from build123d import *

# Parameters (mm, degrees)
EXTRUDE_1_DEPTH     = 2
EXTRUDE_2_DEPTH     = 2
SKETCH_4_R          = 1
CUT_EXTRUDE_1_DEPTH = 2
EXTRUDE_4_DEPTH     = 2
SKETCH_8_R          = 1
CUT_EXTRUDE_3_DEPTH = 2


with BuildPart() as part:
    # 草图1 → 凸台-拉伸1 (new body)
    with BuildSketch(Plane.XY):
        Polygon((27.5, -11.5), (27.5, 11.5), (11.5, 11.5), (11.5, 27.5), (-11.5, 27.5), (-11.5, 11.5), (-27.5, 11.5), (-27.5, -11.5), (-11.5, -11.5), (-11.5, -27.5), (11.5, -27.5), (11.5, -11.5), align=None)
    extrude(amount=EXTRUDE_1_DEPTH)

    # 草图3 → 凸台-拉伸2 (add)
    with BuildSketch(Plane(origin=(0, 27.5, 0), x_dir=(1, 0, 0), z_dir=(0, 1, 0))):
        with BuildLine():
            Line((-11.5, -2), (11.5, -2))
            Line((11.5, -2), (11.5, 19.5))
            ThreePointArc((11.5, 19.5), (0, 31), (-11.5, 19.5))
            Line((-11.5, 19.5), (-11.5, -2))
        make_face()
    extrude_2 = extrude(amount=-EXTRUDE_2_DEPTH)

    # 草图4 → 切除-拉伸1 (cut)
    with BuildSketch(Plane(origin=(0, 27.5, 0), x_dir=(1, 0, 0), z_dir=(0, 1, 0))):
        with Locations((0, 19.5)):
            Circle(SKETCH_4_R)
    cut_extrude_1 = extrude(amount=-CUT_EXTRUDE_1_DEPTH, mode=Mode.SUBTRACT)

    # 镜向2: 凸台-拉伸2, 切除-拉伸1 across plane
    add(extrude_2.mirror(Plane.ZX))
    add(cut_extrude_1.mirror(Plane.ZX), mode=Mode.SUBTRACT)

    # 草图7 → 凸台-拉伸4 (add)
    with BuildSketch(Plane.ZY.offset(27.5)):
        with BuildLine():
            Line((0, 11.5), (21.5, 11.5))
            ThreePointArc((21.5, 11.5), (33, 0), (21.5, -11.5))
            Line((21.5, -11.5), (0, -11.5))
            Line((0, -11.5), (0, 11.5))
        make_face()
    extrude_4 = extrude(amount=-EXTRUDE_4_DEPTH)

    # 草图8 → 切除-拉伸3 (cut)
    with BuildSketch(Plane.ZY.offset(27.5)):
        with Locations((21.5, 0)):
            Circle(SKETCH_8_R)
    cut_extrude_3 = extrude(amount=-CUT_EXTRUDE_3_DEPTH, mode=Mode.SUBTRACT)

    # 镜向4: 凸台-拉伸4, 切除-拉伸3 across plane
    add(extrude_4.mirror(Plane(origin=(0, 0, 0), x_dir=(0, 0, 1), z_dir=(1, 0, 0))))
    add(cut_extrude_3.mirror(Plane(origin=(0, 0, 0), x_dir=(0, 0, 1), z_dir=(1, 0, 0))), mode=Mode.SUBTRACT)


solid = part.part
Geometry: final body of the model. Coordinates: model frame, mm. A direction names the side the tool comes from. Round coordinates to 2 decimals unless told otherwise and drop trailing zeros. Loops run counter-clockwise (first coordinate to the right, second up) from the corner with the lowest first, then second, coordinate; pieces in that order, holes last.
Q1. Access query for faces 1 (the flat face through (-25.5, 0, 18)), 2 (the flat face through (-11.5, -26, -5)), 3 (the flat face through (26, -11.5, 7)), 4 (the flat face through (0, 25.5, -16)), 5 (the flat face through (-11.5, 26, -6)). Directions: +Z, -Z, +X, -X, +Y, -Y. A direction counts if a zero-diameter tool reaches every point of the face in a straight line with its end or side. Return the directions, or none.
Q2. Section B-B on y = 0. Return loops of the section in (x, z).
Q3. Material intervals for L1, parallel to Y at x = 26.25, z = 21.5; L2, parallel to X at y = 1, z = 13, sorted ascending.
Q4. Section A-A on x = 0. Return loops of the section in (y, z), plus the area to 3 significant figures.
Q5. Pin query (flat end, axial travel): P1, Ø1.8, axis at y = 0, z = 21.5, coming from the -X side; P2, Ø13, axis at y = -23, z = -11, coming from the +X side; P3, Ø2, axis at x = -22, y = -2.5, coming from the -Z side; P4, Ø13, axis at x = -20, z = 8, coming from the -Y side. Return the tip coordinate at first contact, or that it passes through.
Q6. Section D-D on y = -16.5. Return loops of the section in (x, z).
Q7. Section C-C on z = -22. Return loops of the section in (x, y), plus the area to 3 significant figures.
Q8. Pull-direction query (X, two-part tool) for faces 6 (the flat face through (11.5, -26, -6)), 7 (the flat face through (26, 11.5, 6)), 8 (the flat face through (25.5, 0, 18)), 9 (the cylindrical face through (-0.217, 26.514, -18.524)); classes: released by +X, released by -X, zero draft, split by the parting line, or undercut.
Evaluation:
1. face 1: +Z, +Y, -Y
1. face 2: +Z, -Z, -X, -Y
1. face 3: +Z, -Z, +X, -Y
1. face 4: -Z, +X, -X
1. face 5: +Z, -Z, -X, +Y
2. outline: (-27.5, 0) - (27.5, 0) - (27.5, 20.5) - (25.5, 20.5) - (25.5, 2) - (-25.5, 2) - (-25.5, 20.5) - (-27.5, 20.5) - close; (-27.5, 22.5) - (-25.5, 22.5) - (-25.5, 33) - (-27.5, 33) - close; (25.5, 22.5) - (27.5, 22.5) - (27.5, 33) - (25.5, 33) - close
3. L1: y = -11.5 to -1, 1 to 11.5
3. L2: x = -27.5 to -25.5, 25.5 to 27.5
4. outline: (-27.5, -31) - (-25.5, -31) - (-25.5, -20.5) - (-27.5, -20.5) - close; (-27.5, -18.5) - (-25.5, -18.5) - (-25.5, 0) - (25.5, 0) - (25.5, -18.5) - (27.5, -18.5) - (27.5, 2) - (-27.5, 2) - close; (25.5, -31) - (27.5, -31) - (27.5, -20.5) - (25.5, -20.5) - close
4. area: 226 mm2
5. P1: passes through
5. P2: stops at x = 11.5
5. P3: stops at z = 0
5. P4: stops at y = -11.5
6. outline: (-11.5, 0) - (11.5, 0) - (11.5, 2) - (-11.5, 2) - close
7. outline: (-11.22, -27.5) - (11.22, -27.5) - (11.22, -25.5) - (-11.22, -25.5) - close; (-11.22, 25.5) - (11.22, 25.5) - (11.22, 27.5) - (-11.22, 27.5) - close
7. area: 89.8 mm2
8. face 6: released by +X
8. face 7: zero draft
8. face 8: undercut
8. face 9: undercut
